```python
from build123d import *

# Parameters (mm, degrees)
SKETCH1_R           = 3.95
BOSS_EXTRUDE1_DEPTH = 5
SKETCH2_R           = 4.4
BOSS_EXTRUDE2_DEPTH = 2
SKETCH4_R           = 2.4
BOSS_EXTRUDE3_DEPTH = 2
BOSS_EXTRUDE4_DEPTH = 6
SKETCH6_R           = 4.4
SKETCH6_R_2         = 3.95
BOSS_EXTRUDE5_DEPTH = 5


with BuildPart() as part:
    # Sketch1 → Boss-Extrude1 (new body)
    with BuildSketch(Plane(origin=(0, 0, 0), x_dir=(1, 0, 0), z_dir=(0, 1, 0))):
        with Locations(Location((0, 0, 0), (0, 0, 270))):
            Circle(SKETCH1_R)
        with BuildLine():
            ThreePointArc((-0.166646614, 2.345141313), (-0.092401566, 2.286261662), (0, 2.2652595))
            ThreePointArc((0, 2.2652595), (0.092401566, 2.286261662), (0.166646614, 2.345141313))
            ThreePointArc((0.166646614, 2.345141313), (0.365153552, 2.422635524), (0.531999564, 2.290073216))
            ThreePointArc((0.531999564, 2.290073216), (0.585591031, 2.211925311), (0.667696959, 2.164620376))
            ThreePointArc((0.667696959, 2.164620376), (0.762183879, 2.157453631), (0.850485509, 2.191833312))
            ThreePointArc((0.850485509, 2.191833312), (1.063015161, 2.207373726), (1.183375246, 2.031522064))
            ThreePointArc((1.183375246, 2.031522064), (1.211551295, 1.941049689), (1.276066113, 1.871645232))
            ThreePointArc((1.276066113, 1.871645232), (1.364242809, 1.836946378), (1.458755034, 1.843771303))
            ThreePointArc((1.458755034, 1.843771303), (1.666423208, 1.795977086), (1.729602845, 1.592461261))
            ThreePointArc((1.729602845, 1.592461261), (1.72985991, 1.497703284), (1.771051193, 1.412366197))
            ThreePointArc((1.771051193, 1.412366197), (1.845082779, 1.353218377), (1.937407773, 1.331882123))
            ThreePointArc((1.937407773, 1.331882123), (2.121762239, 1.225), (2.12214764, 1.011903287))
            ThreePointArc((2.12214764, 1.011903287), (2.094462881, 0.92127937), (2.108670602, 0.827592226))
            ThreePointArc((2.108670602, 0.827592226), (2.161979047, 0.749250985), (2.243913329, 0.701649371))
            ThreePointArc((2.243913329, 0.701649371), (2.388573385, 0.545176288), (2.326130305, 0.341433266))
            ThreePointArc((2.326130305, 0.341433266), (2.272963633, 0.262995741), (2.258925375, 0.169283054))
            ThreePointArc((2.258925375, 0.169283054), (2.286773988, 0.078709355), (2.351037339, 0.009071994))
            ThreePointArc((2.351037339, 0.009071994), (2.443149303, -0.183088729), (2.323426084, -0.3593746))
            ThreePointArc((2.323426084, -0.3593746), (2.249501592, -0.418656214), (2.208464714, -0.504067659))
            ThreePointArc((2.208464714, -0.504067659), (2.208379026, -0.598825947), (2.249261363, -0.68431147))
            ThreePointArc((2.249261363, -0.68431147), (2.280640684, -0.89508551), (2.114275259, -1.028250455))
            ThreePointArc((2.114275259, -1.028250455), (2.026161462, -1.063108727), (1.961772273, -1.13262975))
            ThreePointArc((1.961772273, -1.13262975), (1.933759896, -1.223152935), (1.947628645, -1.316890857))
            ThreePointArc((1.947628645, -1.316890857), (1.915487132, -1.527550015), (1.717261799, -1.605761745))
            ThreePointArc((1.717261799, -1.605761745), (1.622787995, -1.613099364), (1.540767756, -1.660552716))
            ThreePointArc((1.540767756, -1.660552716), (1.487317713, -1.738797417), (1.472940575, -1.832458712))
            ThreePointArc((1.472940575, -1.832458712), (1.380134142, -2.024284997), (1.167662092, -2.040594058))
            ThreePointArc((1.167662092, -2.040594058), (1.075222693, -2.019759044), (0.982859262, -2.040928287))
            ThreePointArc((0.982859262, -2.040928287), (0.908720824, -2.099942118), (0.86737527, -2.185204569))
            ThreePointArc((0.86737527, -2.185204569), (0.722150177, -2.341153374), (0.514310485, -2.294110633))
            ThreePointArc((0.514310485, -2.294110633), (0.432119136, -2.246954269), (0.337619409, -2.239958423))
            ThreePointArc((0.337619409, -2.239958423), (0.249380102, -2.274497747), (0.184739867, -2.343785411))
            ThreePointArc((0.184739867, -2.343785411), (0, -2.45), (-0.184739867, -2.343785411))
            ThreePointArc((-0.184739867, -2.343785411), (-0.249380102, -2.274497747), (-0.337619409, -2.239958423))
            ThreePointArc((-0.337619409, -2.239958423), (-0.432119136, -2.246954269), (-0.514310485, -2.294110633))
            ThreePointArc((-0.514310485, -2.294110633), (-0.722150177, -2.341153374), (-0.86737527, -2.185204569))
            ThreePointArc((-0.86737527, -2.185204569), (-0.908720824, -2.099942118), (-0.982859262, -2.040928287))
            ThreePointArc((-0.982859262, -2.040928287), (-1.075222693, -2.019759044), (-1.167662092, -2.040594058))
            ThreePointArc((-1.167662092, -2.040594058), (-1.380134142, -2.024284997), (-1.472940575, -1.832458712))
            ThreePointArc((-1.472940575, -1.832458712), (-1.487317713, -1.738797417), (-1.540767756, -1.660552716))
            ThreePointArc((-1.540767756, -1.660552716), (-1.622787995, -1.613099364), (-1.717261799, -1.605761745))
            ThreePointArc((-1.717261799, -1.605761745), (-1.915487132, -1.527550015), (-1.947628645, -1.316890857))
            ThreePointArc((-1.947628645, -1.316890857), (-1.933759896, -1.223152935), (-1.961772273, -1.13262975))
            ThreePointArc((-1.961772273, -1.13262975), (-2.026161462, -1.063108727), (-2.114275259, -1.028250455))
            ThreePointArc((-2.114275259, -1.028250455), (-2.280640684, -0.89508551), (-2.249261363, -0.68431147))
            ThreePointArc((-2.249261363, -0.68431147), (-2.208379026, -0.598825947), (-2.208464714, -0.504067659))
            ThreePointArc((-2.208464714, -0.504067659), (-2.249501592, -0.418656214), (-2.323426084, -0.3593746))
            ThreePointArc((-2.323426084, -0.3593746), (-2.443149303, -0.183088729), (-2.351037339, 0.009071994))
            ThreePointArc((-2.351037339, 0.009071994), (-2.286773988, 0.078709355), (-2.258925375, 0.169283054))
            ThreePointArc((-2.258925375, 0.169283054), (-2.272963633, 0.262995741), (-2.326130305, 0.341433266))
            ThreePointArc((-2.326130305, 0.341433266), (-2.388573385, 0.545176288), (-2.243913329, 0.701649371))
            ThreePointArc((-2.243913329, 0.701649371), (-2.161979047, 0.749250985), (-2.108670602, 0.827592226))
            ThreePointArc((-2.108670602, 0.827592226), (-2.094462881, 0.92127937), (-2.12214764, 1.011903287))
            ThreePointArc((-2.12214764, 1.011903287), (-2.121762239, 1.225), (-1.937407773, 1.331882123))
            ThreePointArc((-1.937407773, 1.331882123), (-1.845082779, 1.353218377), (-1.771051193, 1.412366197))
            ThreePointArc((-1.771051193, 1.412366197), (-1.72985991, 1.497703284), (-1.729602845, 1.592461261))
            ThreePointArc((-1.729602845, 1.592461261), (-1.666423208, 1.795977086), (-1.458755034, 1.843771303))
            ThreePointArc((-1.458755034, 1.843771303), (-1.364242809, 1.836946378), (-1.276066113, 1.871645232))
            ThreePointArc((-1.276066113, 1.871645232), (-1.211551295, 1.941049689), (-1.183375246, 2.031522064))
            ThreePointArc((-1.183375246, 2.031522064), (-1.063015161, 2.207373726), (-0.850485509, 2.191833312))
            ThreePointArc((-0.850485509, 2.191833312), (-0.762183879, 2.157453631), (-0.667696959, 2.164620376))
            ThreePointArc((-0.667696959, 2.164620376), (-0.585591031, 2.211925311), (-0.531999564, 2.290073216))
            ThreePointArc((-0.531999564, 2.290073216), (-0.365153552, 2.422635524), (-0.166646614, 2.345141313))
        make_face(mode=Mode.SUBTRACT)
    extrude(amount=BOSS_EXTRUDE1_DEPTH)

    # Sketch2 → Boss-Extrude2 (add)
    with BuildSketch(Plane.XZ):
        with Locations(Location((0, 0, 0), (0, 0, 270))):
            Circle(SKETCH2_R)
    extrude(amount=BOSS_EXTRUDE2_DEPTH)

    # Sketch4 → Boss-Extrude3 (add)
    with BuildSketch(Plane.XZ.offset(2)):
        with Locations(Location((0, 0, 0), (0, 0, 270))):
            Circle(SKETCH4_R)
    extrude(amount=BOSS_EXTRUDE3_DEPTH)

    # Sketch5 → Boss-Extrude4 (add)
    with BuildSketch(Plane.XZ.offset(4)):
        with BuildLine():
            ThreePointArc((1.5, 1.8734994), (0, 2.4), (-1.5, 1.8734994))
            Line((-1.5, 1.8734994), (-1.5, -1.8734994))
            ThreePointArc((-1.5, -1.8734994), (0, -2.4), (1.5, -1.8734994))
            Line((1.5, -1.8734994), (1.5, 1.8734994))
        make_face()
    extrude(amount=BOSS_EXTRUDE4_DEPTH)

    # Sketch6 → Boss-Extrude5 (add)
    with BuildSketch(Plane(origin=(0, 0, 0), x_dir=(1, 0, 0), z_dir=(0, 1, 0))):
        with Locations(Location((0, 0, 0), (0, 0, 270))):
            Circle(SKETCH6_R)
        Circle(SKETCH6_R_2, mode=Mode.SUBTRACT)
    extrude(amount=BOSS_EXTRUDE5_DEPTH)


solid = part.part
```
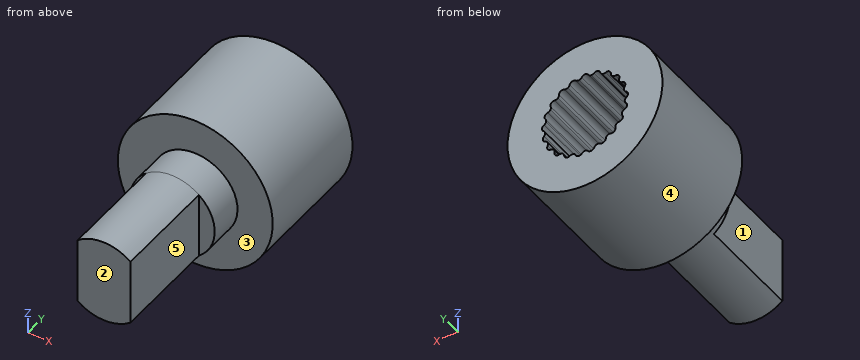
Read the model definition and answer for the solid it produces. Units are mm, in the model's axes. Face numbers are marked on the shaded views. A direction names the side the tool comes from. Coordinates: 2 decimals unless noted, no trailing zeros. Loops run counter-clockwise (first coordinate to the right, second up) from the corner with the lowest first, then second, coordinate; pieces in that order, holes last. Notation, with made-up numbers: (77, 4.25) -> (94, 4.25) arc R19 ccw to (94, 39.25) -> close; hole circle Ø5 at (56.5, -20). An arc over 180 degrees is marked (long way). Return JSON: item names as keys, results as strings.
Item 1: For the marked faces 1, 2, 3, 4 and 5, determine the directions among +Z, -Z, +X, -X, +Y, -Y from which every point of the face is accessible in a straight line to the end or side of a thin tool.
Answers:
{"face 1": "+Z, -Z, -X, -Y", "face 2": "+Z, -Z, +X, -X, -Y", "face 3": "-Y", "face 4": "+Y, -Y", "face 5": "+Z, -Z, +X, -Y"}
Item 2: Find section A-A (z = -0.5). Determine the outline of the cut face in (x, y), plus the area to 3 significant figures.
Answers:
{"outline": "(-4.37, -2) -> (-2.35, -2) -> (-2.35, -4) -> (-1.5, -4) -> (-1.5, -10) -> (1.5, -10) -> (1.5, -4) -> (2.35, -4) -> (2.35, -2) -> (4.37, -2) -> (4.37, 5) -> (2.39, 5) -> (2.39, 0) -> (-2.39, 0) -> (-2.39, 5) -> (-4.37, 5) -> close", "area": "64.7 mm2"}
Item 3: Find section C-C (x = 3.5). Determine the outline of the cut face in (y, z).
Answers:
{"outline": "(-2, -2.67) -> (5, -2.67) -> (5, 2.67) -> (-2, 2.67) -> close"}
Item 4: Find the intervals of material crossed by probe 1 along Z at (x, y) = (-0.5, -5.75); probe 2 along Y at (x, z) = (1.5, -3.75); probe 3 along Y at (x, z) = (0.75, -1), in increasing order.
Answers:
{"probe 1": "z = -2.35 to 2.35", "probe 2": "y = -2 to 5", "probe 3": "y = -10 to 0"}
Item 5: Find section D-D (y = -0.25). Determine the outline of the cut face in (x, z), plus the area to 3 significant figures.
Answers:
{"outline": "circle Ø8.8 at (0, 0)", "area": "60.8 mm2"}
Item 6: Flat-ended cylindrical pins translate along their axes: P1, Ø3, axis at x = -1, y = -7.5, coming from the +Z side; P2, Ø0.7, axis at x = -2, z = 0, coming from the -Y side; P3, Ø1.9, axis at y = -8, z = 0.5, coming from the +X side. Find the tip coordinate at first contact, or state that the pin passes through.
Answers:
{"P1": "stops at z = 2.4", "P2": "stops at y = -4", "P3": "stops at x = 1.5"}
Item 7: Find section B-B (y = -6). Determine the outline of the cut face in (x, z), plus the area to 3 significant figures.
Answers:
{"outline": "(-1.5, -1.87) arc R2.4 ccw to (1.5, -1.87) -> (1.5, 1.87) arc R2.4 ccw to (-1.5, 1.87) -> close", "area": "13.4 mm2"}
